Here's how the part is built. I have some questions about the finished solid (model axes, mm). Face numbers are marked on the shaded views. Round coordinates to 2 decimals unless told otherwise and drop trailing zeros. Loops run counter-clockwise (first coordinate to the right, second up) from the corner with the lowest first, then second, coordinate; pieces in that order, holes last. Notation, with made-up numbers: M 36,-12.5 L 94,-12.5 A12 ccw 94,-7.5 Z; hole C -6,-19.5 d3. An arc over 180 degrees is marked long. Answer as a JSON object with one key per item and string values.
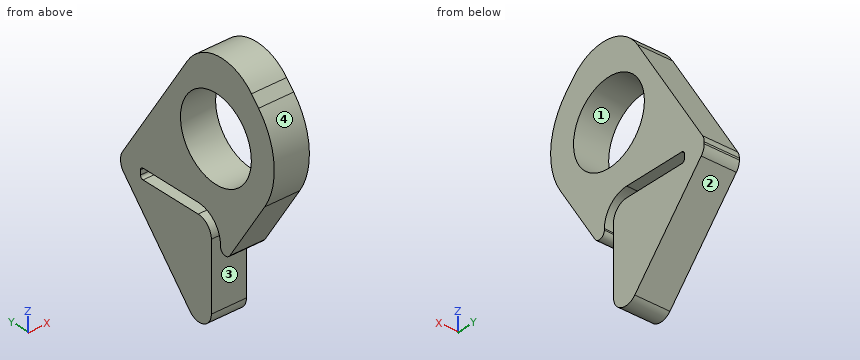
from build123d import *

# Parameters (mm, degrees)
SKETCH3_R           = 3.5
BOSS_EXTRUDE1_DEPTH = 3


with BuildPart() as part:
    # Sketch3 → Boss-Extrude1 (new body)
    with BuildSketch(Plane(origin=(0, 0, 0), x_dir=(0, 0, -1), z_dir=(1, 0, 0))):
        with BuildLine():
            Line((7.72981652, 0.7), (2, 0.7))
            ThreePointArc((2, 0.7), (1.080761184, 1.080761184), (0.7, 2))
            Line((0.7, 2), (0.7, 7.45))
            ThreePointArc((0.7, 7.45), (0.626776695, 7.626776695), (0.45, 7.7))
            Line((0.45, 7.7), (0.05, 7.7))
            ThreePointArc((0.05, 7.7), (-0.126776695, 7.626776695), (-0.2, 7.45))
            Line((-0.2, 7.45), (-0.2, 2))
            ThreePointArc((-0.2, 2), (0.444365081, 0.444365081), (2, -0.2))
            Line((2, -0.2), (2.117066245, -0.2))
            ThreePointArc((2.117066245, -0.2), (2.596969784, -0.559669701), (2.386446273, -1.121229629))
            Line((2.386446273, -1.121229629), (-3.000244885, -4.56606569))
            ThreePointArc((-3.000244885, -4.56606569), (-6.730707864, -5.490615532), (-10.256876598, -3.96179883))
            Line((-10.256876598, -3.96179883), (-11.028611154, -3.264006935))
            ThreePointArc((-11.028611154, -3.264006935), (-12.332100499, 0.034920618), (-10.50093713, 3.072822557))
            Line((-10.50093713, 3.072822557), (-0.446346504, 9.502821112))
            ThreePointArc((-0.446346504, 9.502821112), (-0.188247045, 9.620168933), (0.092413552, 9.660361854))
            Line((0.092413552, 9.660361854), (0.248386958, 9.660361854))
            ThreePointArc((0.248386958, 9.660361854), (0.671058342, 9.583459758), (1.039555867, 9.362610022))
            Line((1.039555867, 9.362610022), (8.520985429, 2.802248168))
            ThreePointArc((8.520985429, 2.802248168), (8.852914424, 1.477328616), (7.72981652, 0.7))
        make_face()
        with Locations((-5.901143056, 0.25)):
            Circle(SKETCH3_R, mode=Mode.SUBTRACT)
    extrude(amount=BOSS_EXTRUDE1_DEPTH)


solid = part.part
Item 1: I want a section at D-D, the plane y = 1. Please give me the cut outline in (x, z), then the cut area to 3 significant figures.
Resolved:
{"outline": "M 0,-8.52 L 3,-8.52 L 3,-1.17 L 0,-1.17 Z; M 0,-0.04 L 3,-0.04 L 3,2.48 L 0,2.48 Z; M 0,9.32 L 3,9.32 L 3,12.13 L 0,12.13 Z", "area": "38.1 mm²"}
Item 2: I want a section at C-C, the plane z = 8. Please give me the cut outline in (x, y), then the cut area to 3 significant figures.
Resolved:
{"outline": "M 0,-5.25 L 3,-5.25 L 3,-2.55 L 0,-2.55 Z; M 0,3.05 L 3,3.05 L 3,4.67 L 0,4.67 Z", "area": "12.9 mm²"}
Item 3: If we mould it in two halves opening along Z, with no side actions, what happens to the marked faces 1, 2, 3 and 4? For each: pulls with the +Z half, pulls with the -Z half, needs draft (parallel to the pull), parting line crosses it, or undercut.
Resolved:
{"face 1": "undercut", "face 2": "pulls with the -Z half", "face 3": "needs draft", "face 4": "parting line crosses it"}
Item 4: I want a section at B-B, the plane y = 4.5. Please give me the cut outline in (x, z).
Resolved:
{"outline": "M 0,-6.58 L 3,-6.58 L 3,-0.7 L 0,-0.7 Z; M 0,0.2 L 3,0.2 L 3,8.27 L 0,8.27 Z"}
Item 5: Please list where these lines run through material, in increasing order: probe 1 along Z at (x, y) = (2.7, 3); probe 2 along Z at (x, y) = (1.95, 2); probe 3 along Y at (x, z) = (2.1, -1.25). Write a range as from..to.
Resolved:
{"probe 1": "-8.3..-0.7, 0.2..3.74, 8.07..10.61", "probe 2": "-8.93..-0.7, 0.2..2.87, 8.93..11.62", "probe 3": "-1.85..-0.07, 0.94..9.18"}
Item 6: I'm going to push flat-ended pins straight in: pin 1 Ø1 at (x, z) = (1.5, -1.5) entering from +Y; pin 2 Ø0.9 at (x, y) = (1.5, 6) entering from -Z; pin 3 Ø1 at (x, z) = (0.5, 4.5) entering from +Y. Where does each tip first touch, or does it pass through?
Resolved:
{"pin 1": "y = 9.4", "pin 2": "z = -5.39", "pin 3": "y = 7.23"}
Item 7: I want a section at A-A, the plane x = 2.2. Please give me the cut outline in (y, z).
Resolved:
{"outline": "M -4.57,3 L -1.12,-2.39 A0.5 ccw -0.2,-2.12 L -0.2,-2 A2.2 cw 2,0.2 L 7.45,0.2 A0.25 cw 7.7,-0.05 L 7.7,-0.45 A0.25 cw 7.45,-0.7 L 2,-0.7 A1.3 ccw 0.7,-2 L 0.7,-7.73 A1.2 ccw 2.8,-8.52 L 9.36,-1.04 A1.2 ccw 9.66,-0.25 L 9.66,-0.09 A1 ccw 9.5,0.45 L 3.07,10.5 A4 ccw -3.26,11.03 L -3.96,10.26 A6 ccw Z; hole C 0.25,5.9 d7"}
